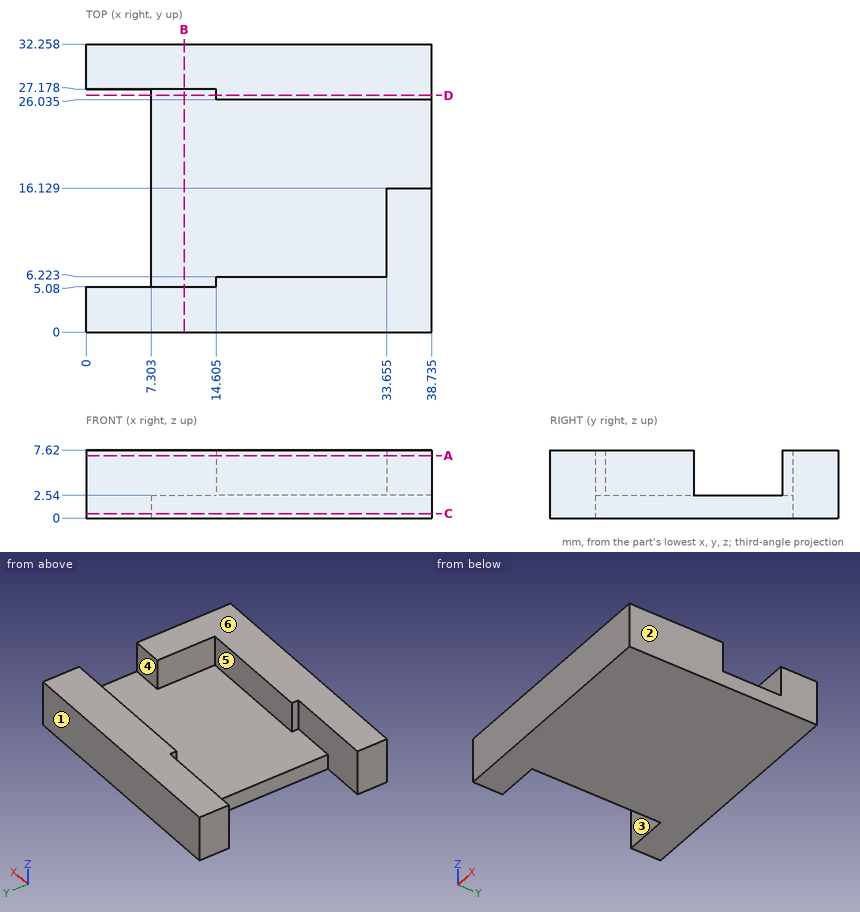
Answer from the drawing. Dimensions are ordinates in mm from the lowest x, y and z of the part. A direction names the side the tool comes from. Coordinates: 2 decimals unless noted, no trailing zeros. Loops run counter-clockwise (first coordinate to the right, second up) from the corner with the lowest first, then second, coordinate; pieces in that order, holes last. Notation, with made-up numbers: (-35.5, 75) - (-2.5, 75) arc R20 ccw to (-2.5, 102) - close; hole circle Ø9 at (-40, 85.25). An arc over 180 degrees is marked (long way). Answer in a Markdown table with one row per item.
1. Find section B-B, the plane x = 11. Write down the section's boundary in (y, z).
Conclusion:
| item | result |
|---|---|
| outline | (0, 0) - (32.26, 0) - (32.26, 7.62) - (27.18, 7.62) - (27.18, 2.54) - (5.08, 2.54) - (5.08, 7.62) - (0, 7.62) - close |
2. Straight lines are drawn through the part: line 1 (Y direction, x = 33, z = 5.75) (1 decimal); line 2 (Y direction, x = 12.5, z = 5.5); line 3 (Z direction, x = 8.5, y = 12). For each, find the intervals that lie inside material, in ascending order.
Conclusion:
| item | result |
|---|---|
| line 1 | y = 0 to 6.2, 26 to 32.3 |
| line 2 | y = 0 to 5.08, 27.18 to 32.26 |
| line 3 | z = 0 to 2.54 |
3. Given pin 1 (11 mm diameter, centred on x = 26.5, y = 15.5, fed in from +Z); pin 2 (0.8 mm diameter, centred on y = 16, z = 1, fed in from -X); pin 3 (1.5 mm diameter, centred on y = 11, z = 5.5, fed in from -X) (1 decimal), each flat-ended and moving along its own axis, determine where each tip first touches the part or whether it passes through.
Conclusion:
| item | result |
|---|---|
| pin 1 | stops at z = 2.54 |
| pin 2 | stops at x = 7.3 |
| pin 3 | stops at x = 33.7 |
4. Find section D-D, the plane y = 26.5. Write down the section's boundary in (x, z) (1 decimal).
Conclusion:
| item | result |
|---|---|
| outline | (7.3, 0) - (38.7, 0) - (38.7, 7.6) - (14.6, 7.6) - (14.6, 2.5) - (7.3, 2.5) - close |
5. Determine the mould class of the marked faces 1, 2, 3 and 4 for opening direction Y: +Y half, -Y half, draft (parallel to the pull), parting line (faces both ways), or undercut.
Conclusion:
| item | result |
|---|---|
| face 1 | +Y half |
| face 2 | draft |
| face 3 | undercut |
| face 4 | undercut |
6. Which of the six approach directions +Z, -Z, +X, -X, +Y, -Y give full straight-line access (tool end or side, diameter ignored) to the marked faces 5 and 6?
Conclusion:
| item | result |
|---|---|
| face 5 | +Z, -X |
| face 6 | +Z, +X, -X, +Y, -Y |
7. Find section C-C, the plane z = 0.5. Write down the section's boundary in (x, y) (1 decimal), then the cut area to 3 significant figures.
Conclusion:
| item | result |
|---|---|
| outline | (0, 0) - (38.7, 0) - (38.7, 32.3) - (0, 32.3) - (0, 27.2) - (7.3, 27.2) - (7.3, 5.1) - (0, 5.1) - close |
| area | 1,090 mm² |
8. Find section A-A, the plane z = 7. Write down the section's boundary in (x, y) (1 decimal), then the cut area to 3 significant figures.
Conclusion:
| item | result |
|---|---|
| outline | (0, 0) - (38.7, 0) - (38.7, 16.1) - (33.7, 16.1) - (33.7, 6.2) - (14.6, 6.2) - (14.6, 5.1) - (0, 5.1) - close; (0, 27.2) - (14.6, 27.2) - (14.6, 26) - (38.7, 26) - (38.7, 32.3) - (0, 32.3) - close |
| area | 499 mm² |
